Input: part model. Units: mm. Frame: model coordinates. Face numbers are marked on the shaded views. Give positions to 0.01 mm unless a question says otherwise; leave off trailing zeros. Loops run counter-clockwise (first coordinate to the right, second up) from the corner with the lowest first, then second, coordinate; pieces in that order, holes last. Notation, with made-up numbers: (18.25, -33.75) - (55.25, -33.75) arc R29 cw to (55.25, -10.75) - close; hole circle Ø2 at (44, -5.5). An arc over 180 degrees is marked (long way). Answer as a JSON object with one key per item and string values.
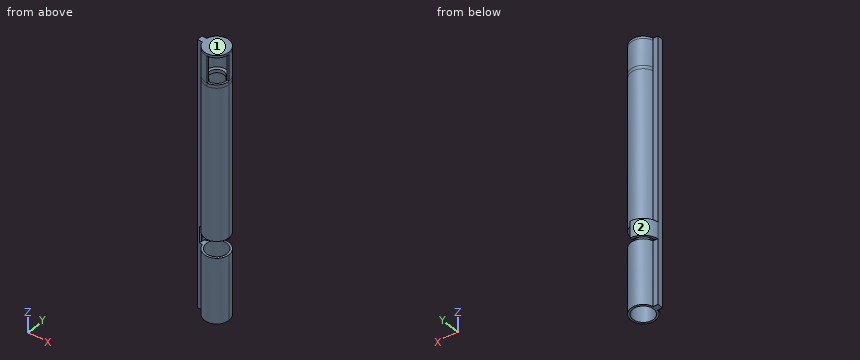
from build123d import *
from build123d.topology import SkipClean

# Parameters (mm, degrees)
SCHIZZO1_R                    = 11
SCHIZZO1_R_2                  = 9.25
TUBO_DEPTH                    = 210
INGRESSOCAVI_DEPTH            = 27
SCHIZZO4_R                    = 11
SCHIZZO4_R_2                  = 6.5
FONDOCORSA_DEPTH              = 3
SCHIZZO5_R                    = 11
TAPPO_DEPTH                   = 2
BASEINFERIORE_DEPTH           = 239
SCHIZZO7_R                    = 13.5
TAGLIOANELLO_DEPTH            = 15
SUPPORTOANELLO_DEPTH          = 15
FACILITAZIONEUSCITACAVI_DEPTH = 3
RACCORDOFACILITAZIONECAVI_R   = 8


with BuildPart() as part:
    # Schizzo1 → Tubo (new body)
    with BuildSketch(Plane.XY):
        Circle(SCHIZZO1_R)
        Circle(SCHIZZO1_R_2, mode=Mode.SUBTRACT)
    extrude(amount=TUBO_DEPTH)

    # Schizzo2 → IngressoCavi (add)
    with BuildSketch(Plane.XY.offset(210)):
        with BuildLine():
            Line((0, -9.25), (0, -11))
            ThreePointArc((0, -11), (-7.778174593, 7.778174593), (11, 0))
            Line((11, 0), (9.25, 0))
            ThreePointArc((9.25, 0), (-6.540737726, 6.540737726), (0, -9.25))
        make_face()
    extrude(amount=INGRESSOCAVI_DEPTH)

    # Schizzo4 → FondoCorsa (add)
    with SkipClean():  # the faces are left unmerged after this step: merging them gives an invalid solid
        with BuildSketch(Plane.XY.offset(210)):
            Circle(SCHIZZO4_R)
            Circle(SCHIZZO4_R_2, mode=Mode.SUBTRACT)
        extrude(amount=FONDOCORSA_DEPTH)

    # Schizzo5 → Tappo (add)
    with SkipClean():  # the faces are left unmerged after this step: merging them gives an invalid solid
        with BuildSketch(Plane.XY.offset(237)):
            Circle(SCHIZZO5_R)
        extrude(amount=TAPPO_DEPTH)
    add(part.part.scale(1), mode=Mode.REPLACE)  # the faces are merged on a copy

    # Schizzo6 → BaseInferiore (add)
    with SkipClean():  # the faces are left unmerged after this step: merging them gives an invalid solid
        with BuildSketch(Plane.XY):
            Polygon((-11, 2.5), (-15, 2.5), (-15, -2.5), (-11, -2.5), (-10.712142643, -2.5), (-10.712142643, 2.5), align=None)
        extrude(amount=BASEINFERIORE_DEPTH)

    # Schizzo7 → TaglioAnello (cut)
    with BuildSketch(Plane.XY.offset(73.5)):
        Circle(SCHIZZO7_R)
    extrude(amount=-TAGLIOANELLO_DEPTH, mode=Mode.SUBTRACT)

    # Schizzo8 → SupportoAnello (add)
    with SkipClean():  # the faces are left unmerged after this step: merging them gives an invalid solid
        with BuildSketch(Plane.XY.offset(73.5)):
            with BuildLine():
                Line((0, 15), (0, 13))
                ThreePointArc((0, 13), (-9.192388155, 9.192388155), (-13, 0))
                Line((-13, 0), (-15, 0))
                ThreePointArc((-15, 0), (-10.606601718, 10.606601718), (0, 15))
            make_face()
        extrude(amount=-SUPPORTOANELLO_DEPTH)

    # Schizzo9 → FacilitazioneUscitaCavi (cut)
    with SkipClean():  # the faces are left unmerged after this step: merging them gives an invalid solid
        with BuildSketch(Plane(origin=(0, 0, 210), x_dir=(-1, 0, 0), z_dir=(0, 0, -1))):
            with BuildLine():
                Line((0, 0), (-9.25, 0))
                ThreePointArc((-9.25, 0), (-6.540737726, -6.540737726), (0, -9.25))
                Line((0, -9.25), (0, 0))
            make_face()
        extrude(amount=-FACILITAZIONEUSCITACAVI_DEPTH, mode=Mode.SUBTRACT)

    # RaccordoFacilitazioneCavi
    # the kernel refuses this fillet: 8 mm, written as the material it takes off along each edge
    with BuildSketch(Plane(origin=(6.5, 0, 201.530207244), x_dir=(1, 0, 0), z_dir=(0, 0, 1)), Plane(origin=(0, -6.5, 221.469792756), x_dir=(0, -1, 0), z_dir=(0, 0, -1))) as raccordofacilitazionecavi_piece_1:
        with BuildLine():
            CenterArc((6.030405405, 7.296501927), RACCORDOFACILITAZIONECAVI_R, 210.212403153, 35.579578639)
            Line((-0.882921715, 3.270845692), (-1.021188257, 3.190332567))
            ThreePointArc((-1.021188257, 3.190332567), (-0.379082322, 1.65226111), (-0.16, 0))
            Line((-0.16, 0), (0, -0.16))
            ThreePointArc((0, -0.16), (1.375, -0.16), (2.684391892, -0.145930039))
            Line((2.684391892, -0.145930039), (2.75, 0))
        make_face()
    extrude(amount=19.939585512, mode=Mode.SUBTRACT)


solid = part.part
Item 1: Contact query for flat-ended pins moving along their axis: P1, Ø12, axis at x = 3, z = 163, coming from the -Y side; P2, Ø5, axis at x = 0.5, y = 4.5, coming from the -Z side; P3, Ø1.4, axis at y = -10.5, z = 228, coming from the +X side; P4, Ø2, axis at x = -13, z = 168.5, coming from the -Y side. Output: stop coordinate, or through.
Geometry check:
{"P1": "stops at y = -11", "P2": "stops at z = 210", "P3": "stops at x = 0", "P4": "stops at y = -2.5"}
Item 2: Material intervals for line 1 (X direction, y = 0, z = 212.05); line 2 (Z direction, x = 2, y = 6.75); line 3 (Z direction, x = -7.5, y = 6), sorted ascending. Write a range as [from, to].
Geometry check:
{"line 1": "x = [-15, -6.5], [9.25, 11]", "line 2": "z = [210, 213], [237, 239]", "line 3": "z = [0, 58.5], [73.5, 239]"}
Item 3: Mould query, pull axis Z, two halves, no side actions, for the marked faces 1 and 2. Classes: released by +Z, released by -Z, zero draft, split by the parting line, or undercut.
Geometry check:
{"face 1": "released by +Z", "face 2": "zero draft"}
Item 4: Cut plane A-A (z = 137.5). Return loops of the section in (x, y), then the cut area to 3 significant figures.
Geometry check:
{"outline": "(-15, -2.5) - (-10.71, -2.5) arc R11 ccw (long way) to (-10.71, 2.5) - (-15, 2.5) - close; hole circle Ø18.5 at (0, 0)", "area": "132 mm2"}
